Could you check a few things on this model? Use its own coordinates, in mm. Face numbers are marked on the shaded views. A direction names the side the tool comes from. Coordinates: 2 decimals unless noted, no trailing zeros. Order: outer loops, then holes, each group sorted by start corner. A loop starts at its lowest first (then second) coordinate and runs counter-clockwise, first axis right, second up. Notation, with made-up numbers: (-17.5, 2) - (8.5, 2) arc R21 ccw to (8.5, 39) - close; hole circle Ø9 at (68, 29.5). An arc over 180 degrees is marked (long way). Answer as a JSON object with one key per item and string values. Group by question number.
(1) We'd pull the mould along Y, two halves only. Please class the marked faces 1, 2, 3 and 4: pulls with the +Y half, pulls with the -Y half, needs draft (parallel to the pull), parting line crosses it, or undercut.
(2) Imagine slicing it at D-D, the plane x = 29. Write out the boundary of the cut face in (y, z) (3 decimals).
(3) Imagine slicing it at A-A, the plane z = -26. Write out the boundary of the cut face in (x, y) (3 decimals), and give its area (3 significant figures).
(4) Will these pins go through, and if not, where does the flat tip stop? P1, Ø10, axis at y = 37, z = -9, coming from the -X side; P2, Ø8, axis at y = 37.5, z = -14, coming from the +X side.
(5) Please list where these lines run through material, in increasing order: probe 1 along Y at (x, z) = (22.5, -39.5) (3 decimals); probe 2 along Z at (x, y) = (5.5, 36.5) (3 decimals); probe 3 along X at (y, z) = (3, -40.5).
(6) Which directions (+Z, -Z, +X, -X, +Y, -Y) give clear straight access to the entire face, cutting with the end or side of a thin tool? Please do the marked faces 5 and 6.
(7) Imagine slicing it at B-B, the plane x = 15. Write out the boundary of the cut face in (y, z) (3 decimals), and give its area (3 significant figures).
(8) Imagine slicing it at C-C, the plane y = 27. Write out the boundary of the cut face in (x, z) (3 decimals), and give its area (3 significant figures).
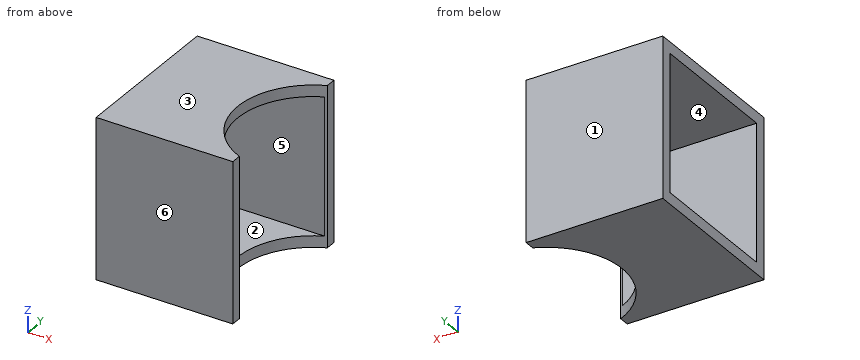
from build123d import *

# Parameters (mm, degrees)
SKETCH1_W               = 44.45
SKETCH1_H               = 44.45
SKETCH1_W_2             = 38.1
SKETCH1_H_2             = 38.1
BOSS_EXTRUDE1_DEPTH     = 38.1
SKETCH2_R               = 21.082
CUT_EXTRUDE1_DEPTH      = 1
CUT_EXTRUDE1_DEPTH_BACK = 45.45


with BuildPart() as part:
    # Sketch1 → Boss-Extrude1 (new body)
    with BuildSketch(Plane(origin=(0, 0, 0), x_dir=(0, 0, -1), z_dir=(1, 0, 0))):
        with Locations((22.225, 22.225)):
            Rectangle(SKETCH1_W, SKETCH1_H)
        with Locations((22.225, 22.225)):
            Rectangle(SKETCH1_W_2, SKETCH1_H_2, mode=Mode.SUBTRACT)
    extrude(amount=BOSS_EXTRUDE1_DEPTH)

    # Sketch2 → Cut-Extrude1 (cut, two sides)
    with BuildSketch(Plane.XY) as cut_extrude1_sk:
        with Locations((46.482, 22.225)):
            Circle(SKETCH2_R)
    extrude(amount=CUT_EXTRUDE1_DEPTH, mode=Mode.SUBTRACT)
    extrude(cut_extrude1_sk.sketch, amount=-CUT_EXTRUDE1_DEPTH_BACK, mode=Mode.SUBTRACT)


solid = part.part
Result set:
{
 "1": {"face 1": "pulls with the +Y half", "face 2": "undercut", "face 3": "needs draft", "face 4": "undercut"},
 "2": {"outline": "(0, -44.45) - (10.442, -44.45) - (10.442, -41.275) - (3.175, -41.275) - (3.175, -3.175) - (10.442, -3.175) - (10.442, 0) - (0, 0) - close; (34.008, -44.45) - (44.45, -44.45) - (44.45, 0) - (34.008, 0) - (34.008, -3.175) - (41.275, -3.175) - (41.275, -41.275) - (34.008, -41.275) - close"},
 "3": {"outline": "(0, 0) - (38.1, 0) - (38.1, 2.881) arc R21.082 cw to (37.452, 3.175) - (0, 3.175) - close; (0, 41.275) - (37.452, 41.275) arc R21.082 cw to (38.1, 41.569) - (38.1, 44.45) - (0, 44.45) - close", "area": "242 mm^2"},
 "4": {"P1": "stops at x = 0", "P2": "stops at x = 37.94"},
 "5": {"probe 1": "y = 0 to 3.175, 41.275 to 44.45", "probe 2": "z = -44.45 to -41.275, -3.175 to 0", "probe 3": "x = 0 to 37.83"},
 "6": {"face 5": "+X, -X", "face 6": "+Z, -Z, +X, -X, -Y"},
 "7": {"outline": "(0, -44.45) - (44.45, -44.45) - (44.45, 0) - (0, 0) - close; hole (3.175, -41.275) - (41.275, -41.275) - (41.275, -3.175) - (3.175, -3.175) - close", "area": "524 mm^2"},
 "8": {"outline": "(0, -44.45) - (25.948, -44.45) - (25.948, -41.275) - (0, -41.275) - close; (0, -3.175) - (25.948, -3.175) - (25.948, 0) - (0, 0) - close", "area": "165 mm^2"}
}
